```python
from build123d import *

# Parameters (mm, degrees)
F1_DEPTH = 25
F2_DEPTH = 5
F3_R     = 4.99999
F4_R     = 1


# Not quite as in the source:
# - a fillet or chamfer is up to 0.001 mm smaller than in the source, because OpenCascade refuses the exact size


with BuildPart() as f1:
    # F0 (on Front) → F1 (new body, symmetric)
    with BuildSketch(Plane.XZ):
        Polygon((4.6798147489, 17.465306413), (0, 0), (-11.1081470023, 2.9764190187), (-7.2258613258, 17.465306413), (-9.2258613258, 17.465306413), (-13.9056760747, 0), (-14.4415744596, -2), (1.4641016151, -2), (4.071958182, 7.7326532065), (6.6798147489, 17.465306413), align=None)
    extrude(amount=F1_DEPTH, both=True)

    # F0 (on Front) → F2 (join, symmetric)
    with BuildSketch(Plane.XZ):
        Polygon((31.4641016151, -2), (4.071958182, 7.7326532065), (1.4641016151, -2), align=None)
    extrude(amount=F2_DEPTH, both=True)

    # F3 (radius 5 in the source; OpenCascade refuses exactly that, so slightly less here)
    f3_edges = [f1.edges().sort_by_distance(p)[0] for p in [
        (2.76803, -5, 2.866327),
        (4.071958, 0, 7.732653),
        (2.76803, 5, 2.866327),
        (17.76803, 5, 2.866327),
        (17.76803, -5, 2.866327),
        (5.679815, -25, 17.465306),
        (-8.225861, -25, 17.465306),
        (-8.225861, 25, 17.465306),
        (5.679815, 25, 17.465306),
    ]]
    fillet(f3_edges, radius=F3_R)

    # F4
    f4_edges = [f1.edges().sort_by_distance(p)[0] for p in [
        (-9.225861, 0, 17.465306),
        (6.679815, 0, 17.465306),
    ]]
    fillet(f4_edges, radius=F4_R)


solid = f1.part
```
Input: part model. Units: mm. Frame: model coordinates. A direction names the side the tool comes from. Give positions to 0.01 mm unless a question says otherwise; leave off trailing zeros. Write each loop counter-clockwise with the first axis right and the second up, starting at its lowest first coordinate (ties: lowest second). Pieces come first, ordered by that corner, then holes. Notation, with made-up numbers: (-31.5, 47) - (-5.5, 47) arc R20 cw to (-5.5, 69) - close; hole circle Ø1 at (-37.75, 86.25). An arc over 180 degrees is marked (long way). Write item = value, one per line. Start each with the question number.
1. Mould query, pull axis Z, two halves, no side actions, for faces 3 (the flat face through (-6, -25, 1)), 4 (the cylindrical face through (3.44, -6.5, -0.15)), 5 (the flat face through (-9.2, -0.4, 10.1)), 6 (the cylindrical face through (-8.394, -23.574, 15.962)). Classes: released by +Z, released by -Z, zero draft, split by the parting line, or undercut.
2. Ray query, L1, parallel to X at y = -14.5, z = 14; L2, parallel to X at y = 2.5, z = 7.5; L3, parallel to Y at x = 12, z = -0.5. Return the intervals inside material, ascending.
3. Section query A-A, the plane y = 17.5. Output: boundary loops of the cut face in (x, z), then the cut area to 3 significant figures.
4. Access query for faces 1 (the flat face through (2.37, -0.35, 8.85)), 2 (the flat face through (-5.48, -0.35, 1.47)). Directions: +Z, -Z, +X, -X, +Y, -Y. A direction counts if a zero-diameter tool reaches every point of the face in a straight line with its end or side. Return the directions, or none.
5. First-contact query: pin 1 Ø6 at (x, z) = (1, 14.5) entering from -Y; pin 2 Ø3 at (x, z) = (9.5, 2) entering from +Y; pin 3 Ø4 at (y, z) = (-0.5, 11) entering from -X. Flat tips, straight axial feed; report the tip coordinate or a pass-through.
6. Section query B-B, the plane x = -2. Output: boundary loops of the cut face in (y, z).
Check sheet entries:
q1.face_3 = zero draft
q1.face_4 = released by -Z
q1.face_5 = undercut
q1.face_6 = released by +Z
q2.L1 = -10.15 to -8.15, 3.75 to 5.75
q2.L2 = -11.9 to -9.9, 2.01 to 5.87
q2.L3 = -5 to 5
q3.outline = (-14.44, -2) - (1.46, -2) - (6.34, 16.21) arc R1 ccw to (5.38, 17.47) - (4.68, 17.47) - (0, 0) - (-11.11, 2.98) - (-7.23, 17.47) - (-8.46, 17.47) arc R1 ccw to (-9.42, 16.72) - close
q3.area = 119 mm2
q4.face_1 = +Z, +Y, -Y
q4.face_2 = +Y, -Y
q5.pin_1 = -24.99
q5.pin_2 = 5
q5.pin_3 = -11.49
q6.outline = (-25, -2) - (25, -2) - (25, 0.54) - (-25, 0.54) - close
